Design review of the part built by this model. Coordinates are the model's own, in mm. Face numbers are marked on the shaded views. A direction names the side the tool comes from. Give positions to 0.01 mm unless a question says otherwise; leave off trailing zeros. Write each loop counter-clockwise with the first axis right and the second up, starting at its lowest first coordinate (ties: lowest second). Pieces come first, ordered by that corner, then holes. Notation, with made-up numbers: M -5,82.25 L 14,82.25 A37 ccw 14,121.25 Z; hole C 28.5,47 d10. An arc over 180 degrees is marked long. One line per item, written item: value. Start each with the question number.
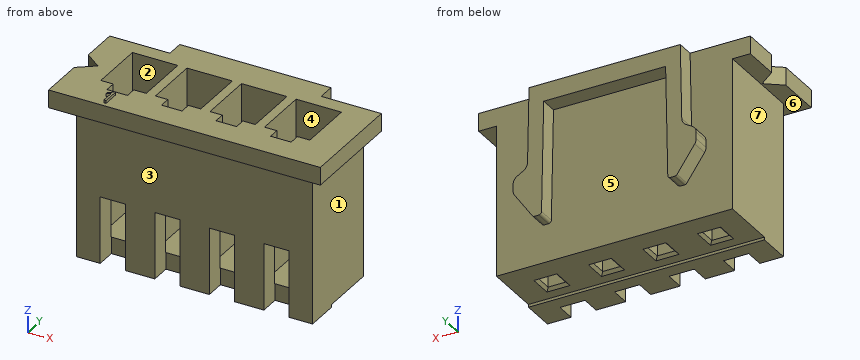
```python
from build123d import *

# Parameters (mm, degrees)
SKETCH1_W                   = 10.7696
SKETCH1_H                   = 4.0894
BODY_DEPTH                  = 7.6962
FLANGE_DEPTH                = 0.8128
LOCK_DEPTH                  = 0.7874
SKETCH4_W                   = 2.0701
SKETCH4_H                   = 2.54
PIN_CAVITY_DEPTH            = 7.0612
SKETCH5_W                   = 0.8001
SKETCH5_H                   = 0.8001
PIN_ENTRY_DEPTH             = 0.635
SKETCH6_W                   = 0.9398
SKETCH6_H                   = 0.508
PIN_LOCK_DEPTH              = 3.175
SKETCH8_W                   = 10.7696
SKETCH8_H                   = 1.524
BODY_EXTEND_DEPTH           = 0.127
SKETCH7_W                   = 1.143
SKETCH7_H                   = 3.048
PIN_CAV_CUTOUT_DEPTH        = 0.889
CHAMFER1_SIZE               = 0.127
F_4_POSITION_COUNT          = 4
F_4_POSITION_PITCH          = 2.4892
CHAMFER1_OF_4_POSITION_SIZE = 0.127
PIN_1_INDICATOR_REACH       = 9.823
PIN_NUMBER_DEPTH            = 0.127


with BuildPart() as part:
    # Sketch1 → BODY (new body)
    with BuildSketch(Plane.XY):
        Rectangle(SKETCH1_W, SKETCH1_H)
    extrude(amount=-BODY_DEPTH)

    # Sketch2 → FLANGE (add)
    with BuildSketch(Plane.XY):
        Polygon((5.3848, -2.0447), (5.3848, 2.0447), (6.1976, 2.0447), (6.1976, -2.8575), (-6.1976, -2.8575), (-6.1976, 2.0447), (-5.3848, 2.0447), (-5.3848, -2.0447), align=None)
    extrude(amount=-FLANGE_DEPTH)

    # Sketch3 → LOCK (add)
    with BuildSketch(Plane(origin=(0, 2.0447, 0), x_dir=(-1, 0, 0), z_dir=(0, 1, 0))):
        with BuildLine():
            Line((-3.451217359, 0), (-3.518566627, -3.417975309))
            ThreePointArc((-3.518566627, -3.417975309), (-3.571148904, -3.603734382), (-3.708036257, -3.739871011))
            Line((-3.708036257, -3.739871011), (-3.988756426, -3.903032559))
            ThreePointArc((-3.988756426, -3.903032559), (-4.12753166, -4.042413008), (-4.1783, -4.232434193))
            Line((-4.1783, -4.232434193), (-4.1783, -4.529184562))
            ThreePointArc((-4.1783, -4.529184562), (-4.160969658, -4.642786409), (-4.110555225, -4.746053564))
            Line((-4.110555225, -4.746053564), (-3.301776384, -5.914289667))
            ThreePointArc((-3.301776384, -5.914289667), (-3.256299524, -5.954493973), (-3.197357976, -5.969))
            Line((-3.197357976, -5.969), (-3.007422189, -5.969))
            ThreePointArc((-3.007422189, -5.969), (-2.918508611, -5.932682829), (-2.880446837, -5.844501977))
            Line((-2.880446837, -5.844501977), (-2.7813, -0.8128))
            Line((-2.7813, -0.8128), (2.7813, -0.8128))
            Line((2.7813, -0.8128), (2.880446837, -5.844501977))
            ThreePointArc((2.880446837, -5.844501977), (2.918508611, -5.932682829), (3.007422189, -5.969))
            Line((3.007422189, -5.969), (3.197357976, -5.969))
            ThreePointArc((3.197357976, -5.969), (3.256299524, -5.954493973), (3.301776384, -5.914289667))
            Line((3.301776384, -5.914289667), (4.110555225, -4.746053564))
            ThreePointArc((4.110555225, -4.746053564), (4.160969658, -4.642786409), (4.1783, -4.529184562))
            Line((4.1783, -4.529184562), (4.1783, -4.232434193))
            ThreePointArc((4.1783, -4.232434193), (4.12753166, -4.042413008), (3.988756426, -3.903032559))
            Line((3.988756426, -3.903032559), (3.708036257, -3.739871011))
            ThreePointArc((3.708036257, -3.739871011), (3.571148904, -3.603734382), (3.518566627, -3.417975309))
            Line((3.518566627, -3.417975309), (3.451217359, 0))
            Line((3.451217359, 0), (-3.451217359, 0))
        make_face()
    extrude(amount=LOCK_DEPTH)

    # Sketch4 → PIN CAVITY (cut)
    with BuildSketch(Plane.XY):
        with Locations((-3.7338, 0.0889)):
            Rectangle(SKETCH4_W, SKETCH4_H)
    pin_cavity = extrude(amount=-PIN_CAVITY_DEPTH, mode=Mode.SUBTRACT)

    # Sketch5 → PIN ENTRY (cut)
    with BuildSketch(Plane.XY.offset(-7.0612)):
        with Locations((-3.7338, 0.4953)):
            Rectangle(SKETCH5_W, SKETCH5_H)
    pin_entry = extrude(amount=-PIN_ENTRY_DEPTH, mode=Mode.SUBTRACT)

    # Sketch6 → PIN LOCK (cut)
    with BuildSketch(Plane.XY):
        with Locations((-3.7338, -1.4351)):
            Rectangle(SKETCH6_W, SKETCH6_H)
    pin_lock = extrude(amount=-PIN_LOCK_DEPTH, mode=Mode.SUBTRACT)

    # Sketch8 → BODY EXTEND (add)
    with BuildSketch(Plane(origin=(0, 0, -7.6962), x_dir=(-1, 0, 0), z_dir=(0, 0, -1))):
        with Locations((0, -1.2827)):
            Rectangle(SKETCH8_W, SKETCH8_H)
    extrude(amount=BODY_EXTEND_DEPTH)

    # Sketch7 → PIN CAV CUTOUT (cut)
    with BuildSketch(Plane.XZ.offset(2.0447)):
        with Locations((-3.7338, -6.2992)):
            Rectangle(SKETCH7_W, SKETCH7_H)
    pin_cav_cutout = extrude(amount=-PIN_CAV_CUTOUT_DEPTH, mode=Mode.SUBTRACT)

    # Chamfer1
    chamfer1_edges = [part.edges().sort_by_distance(p)[0] for p in [
        (-3.7338, 0.09525, -7.6962),
        (-4.13385, 0.4953, -7.6962),
        (-3.7338, 0.89535, -7.6962),
        (-3.33375, 0.4953, -7.6962),
    ]]
    chamfer(chamfer1_edges, length=CHAMFER1_SIZE)

    # 4 POSITION: PIN CAVITY, PIN ENTRY, PIN LOCK, PIN CAV CUTOUT ×4
    with Locations(*[(i * F_4_POSITION_PITCH, 0, 0) for i in range(1, F_4_POSITION_COUNT)]):
        add(pin_cavity, mode=Mode.SUBTRACT)
        add(pin_entry, mode=Mode.SUBTRACT)
        add(pin_lock, mode=Mode.SUBTRACT)
        add(pin_cav_cutout, mode=Mode.SUBTRACT)

    # Chamfer1 of 4 POSITION
    chamfer1_of_4_position_edges = [part.edges().sort_by_distance(p)[0] for p in [
        (-1.2446, 0.09525, -7.6962),
        (-1.64465, 0.4953, -7.6962),
        (-1.2446, 0.89535, -7.6962),
        (-0.84455, 0.4953, -7.6962),
        (1.2446, 0.09525, -7.6962),
        (0.84455, 0.4953, -7.6962),
        (1.2446, 0.89535, -7.6962),
        (1.64465, 0.4953, -7.6962),
        (3.7338, 0.09525, -7.6962),
        (3.33375, 0.4953, -7.6962),
        (3.7338, 0.89535, -7.6962),
        (4.13385, 0.4953, -7.6962),
    ]]
    chamfer(chamfer1_of_4_position_edges, length=CHAMFER1_OF_4_POSITION_SIZE)

    # Sketch9 → PIN 1 INDICATOR (cut, up to next)
    with BuildSketch(Plane.XY, mode=Mode.PRIVATE) as pin_1_indicator_sk1:
        Polygon((-6.1976, 0.3302), (-5.4356, -0.2413), (-6.1976, -0.8128), align=None)
    pin_1_indicator_tool1 = extrude(pin_1_indicator_sk1.sketch, amount=-PIN_1_INDICATOR_REACH, mode=Mode.PRIVATE) & part.part
    add(pin_1_indicator_tool1.solids().sort_by_distance((-5.9436, -0.2413, 0))[0], mode=Mode.SUBTRACT)

    # Sketch10 → PIN NUMBER (add)
    with BuildSketch(Plane.XY):
        with BuildLine():
            Line((-3.692543038, -2.6543), (-3.791324526, -2.6543))
            Line((-3.791324526, -2.6543), (-3.791324526, -2.053893769))
            add(Edge.make_bspline(
                [(-3.791324526, -2.053893769), (-3.797012373, -2.059378997), (-3.808833939, -2.070779444), (-3.828817048, -2.086913922), (-3.851120752, -2.103266899), (-3.875455422, -2.118992116), (-3.900260501, -2.133795711), (-3.924231417, -2.147109269), (-3.946967964, -2.158375769), (-3.961944651, -2.164536336), (-3.969131205, -2.16749248)],
                knots=[0, 0, 0, 0, 2.3696e-05, 4.9249e-05, 7.6971e-05, 0.000106639, 0.000136126, 0.000163621, 0.000188885, 0.000212192, 0.000212192, 0.000212192, 0.000212192], degree=3))
            Line((-3.969131205, -2.16749248), (-3.969131205, -2.076428296))
            add(Edge.make_bspline(
                [(-3.969131205, -2.076428296), (-3.956787556, -2.070071292), (-3.932458956, -2.057542014), (-3.898087905, -2.035902229), (-3.865998831, -2.012443811), (-3.836722936, -1.987171954), (-3.810478961, -1.96133958), (-3.788362783, -1.935273699), (-3.769857373, -1.909929775), (-3.760572857, -1.892255199), (-3.756133621, -1.883804395)],
                knots=[0, 0, 0, 0, 4.1637e-05, 8.2064e-05, 0.000121702, 0.000160776, 0.000197993, 0.000232045, 0.000263265, 0.000291868, 0.000291868, 0.000291868, 0.000291868], degree=3))
            Line((-3.756133621, -1.883804395), (-3.692543038, -1.883804395))
            Line((-3.692543038, -1.883804395), (-3.692543038, -2.6543))
        make_face()
    extrude(amount=PIN_NUMBER_DEPTH)


solid = part.part
```
Q1. Take a section at B-B, the plane x = 0.5. Give the boundary of the cut face in (y, z), then the cut area to 3 significant figures.
Q2. For P1, Ø0.6, axis at y = 0.5, z = -7, coming from the -X side; P2, Ø2, axis at x = -0.5, z = -3.5, coming from the -Y side; P3, Ø3, axis at y = 0.5, z = -5, coming from the +X side, all flat-tipped, find the tip position at first contact; note any pin that passes through.
Q3. Take a section at C-C, the plane x = -2.5. Give the boundary of the cut face in (y, z), then the cut area to 3 significant figures.
Q4. Take a section at A-A, the plane y = 1.7. Give the boundary of the cut face in (x, z).
Q5. Take a section at D-D, the plane z = -2.5. State how many separate pieces and enclosed holes the cut face has, then the cut area to 3 significant figures.
Q6. Machinability: for the marked faces 1, 2 and 3, which of the approach directions +Z, -Z, +X, -X, +Y, -Y give a long, thin tool a straight path to every point of the face, cutting with its end or side? Answer none if there is none.
Q7. The part is to be moulded in two halves that separate along X. For the marked faces 4, 5, 6 and 7, say which applies: pulls with the +X half, pulls with the -X half, needs draft (parallel to the pull), parting line crosses it, or undercut.
Q8. Wall thickness on line 1 (X direction, y = -0.4, z = -2.75); line 2 (X direction, y = -1.4, z = -2); line 3 (Y direction, x = 1.75, z = -1.75): over which ranges is each line inside the solid? List them lowest first. Write a range as from..to.
Results list:
1. outline: M -2.86,-0.81 L -2.04,-0.81 L -2.04,-7.82 L -0.52,-7.82 L -0.52,-7.7 L 2.04,-7.7 L 2.04,-0.81 L 2.83,-0.81 L 2.83,0 L 1.36,0 L 1.36,-7.06 L -1.18,-7.06 L -1.18,0 L -2.86,0 Z
1. area: 15.0 mm^2
2. P1: stops at x = -5.38
2. P2: stops at y = -2.04
2. P3: stops at x = 5.38
3. outline: M -2.86,-0.81 L -2.04,-0.81 L -2.04,-7.82 L -0.52,-7.82 L -0.52,-7.7 L 2.04,-7.7 L 2.04,-0.81 L 2.83,-0.81 L 2.83,0 L -2.86,0 Z
3. area: 33.0 mm^2
4. outline: M -6.2,-0.81 L -5.38,-0.81 L -5.38,-7.7 L 5.38,-7.7 L 5.38,-0.81 L 6.2,-0.81 L 6.2,0 L -6.2,0 Z
5. separate pieces: 1
5. enclosed holes: 4
5. area: 22.2 mm^2
6. face 1: -Z, +X, +Y, -Y
6. face 2: +Z
6. face 3: -Z, +X, -X, -Y
7. face 4: undercut
7. face 5: undercut
7. face 6: needs draft
7. face 7: pulls with the -X half
8. line 1: x = -5.38..-4.77, -2.7..-2.28, -0.21..0.21, 2.28..2.7, 4.77..5.38
8. line 2: x = -5.38..-4.2, -3.26..-1.71, -0.77..0.77, 1.71..3.26, 4.2..5.38
8. line 3: y = -2.04..-1.18, 1.36..2.04
